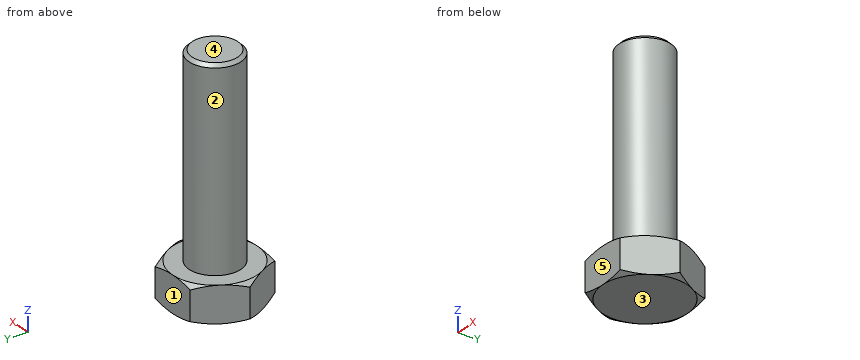
```python
from build123d import *

# Parameters (mm, degrees)
PAD008_DEPTH = 5.5
SKETCH029_R  = 4
PAD009_DEPTH = 30


with BuildPart() as part:
    # Sketch028 → Pad008 (new body)
    with BuildSketch(Plane.XY):
        Polygon((7.5055534995, 0), (3.7527767497, 6.5), (-3.7527767497, 6.5), (-7.5055534995, 0), (-3.7527767497, -6.5), (3.7527767497, -6.5), align=None)
    extrude(amount=PAD008_DEPTH)

    # Sketch029 (on Face8 of Pad008) → Pad009 (join)
    with BuildSketch(Plane.XY.offset(5.5)):
        Circle(SKETCH029_R)
    extrude(amount=PAD009_DEPTH)

    # Sketch030 → Groove001 (revolve, cut)
    with BuildSketch(Plane.XZ):
        Polygon((4, 35.5), (3.5, 35.5), (4, 35), align=None)
        Polygon((7.5055534995, 5.5), (6.5055534995, 5.5), (7.5055534995, 5), align=None)
        Polygon((7.5055534995, 0), (6.5055534995, 0), (7.5055534995, 0.5), align=None)
    revolve(axis=Axis((0, 0, 0), (0, 0, 1)), mode=Mode.SUBTRACT)


solid = part.part
```
Input: part model. Units: mm. Frame: model coordinates. Face numbers are marked on the shaded views. A direction names the side the tool comes from. Round coordinates to 2 decimals unless told otherwise and drop trailing zeros. Loops run counter-clockwise (first coordinate to the right, second up) from the corner with the lowest first, then second, coordinate; pieces in that order, holes last.
1) Set-up query: the marked faces 1 and 2. Return all of +Z, -Z, +X, -X, +Y, -Y with unobstructed straight access to the full face (end or side cutting, diameter ignored); none if empty.
Ans:
face 1: +Z, -Z, +X, -X, +Y
face 2: +Z
2) Pin query (flat end, axial travel): pin 1 (1 mm diameter, centred on x = 0, z = 32, fed in from -Y); pin 2 (6 mm diameter, centred on y = 3.5, z = 26.5, fed in from -X); pin 3 (8 mm diameter, centred on x = -1, z = 25.5, fed in from +Y). Return the tip coordinate at first contact, or that it passes through.
Ans:
pin 1: stops at y = -4
pin 2: stops at x = -3.97
pin 3: stops at y = 4
3) Material intervals for line 1 (Y direction, x = -0.25, z = 24.5); line 2 (Z direction, x = -3.5, y = -2.75); line 3 (X direction, y = 3.5, z = 19.5), sorted ascending.
Ans:
line 1: y = -3.99 to 3.99
line 2: z = 0 to 5.5
line 3: x = -1.94 to 1.94
4) Section query A-A on z = 28. Return the cut outline in (x, y).
Ans:
outline: circle Ø8 at (0, 0)
5) Pull-direction query (Z, two-part tool) for the marked faces 3, 4 and 5; classes: released by +Z, released by -Z, zero draft, split by the parting line, or undercut.
Ans:
face 3: released by -Z
face 4: released by +Z
face 5: zero draft
